```python
from build123d import *

# Parameters (mm, degrees)
SKETCH_2_W               = 22
SKETCH_2_H               = 31.71
EXTRUDE_1_DEPTH          = 22
SKETCH_1_R               = 2.235222544
CUT_EXTRUDE_1_DEPTH      = 38.979461569
CUT_EXTRUDE_2_DEPTH      = 46.024794997
CUT_EXTRUDE_2_DEPTH_BACK = 46.024794997
SKETCH_3_R               = 2.55


with BuildPart() as part:
    # Эскиз2 → Бобышка-Вытянуть1 (new body)
    with BuildSketch(Plane.XY):
        with BuildLine():
            Line((-4.114082915, 26.355832174), (3.885917085, 26.355832174))
            ThreePointArc((3.885917085, 26.355832174), (10.956984897, 23.426899986), (13.885917085, 16.355832174))
            Line((13.885917085, 16.355832174), (13.885917085, -17.554167826))
            ThreePointArc((13.885917085, -17.554167826), (10.956984897, -24.625235638), (3.885917085, -27.554167826))
            Line((3.885917085, -27.554167826), (-4.114082915, -27.554167826))
            ThreePointArc((-4.114082915, -27.554167826), (-11.185150727, -24.625235638), (-14.114082915, -17.554167826))
            Line((-14.114082915, -17.554167826), (-14.114082915, 16.355832174))
            ThreePointArc((-14.114082915, 16.355832174), (-11.185150727, 23.426899986), (-4.114082915, 26.355832174))
        make_face()
        with Locations((-0.114082915, -0.599167826)):
            Rectangle(SKETCH_2_W, SKETCH_2_H, mode=Mode.SUBTRACT)
    extrude(amount=EXTRUDE_1_DEPTH)

    # Эскиз1 → Вырез-Вытянуть1 (cut, through all)
    with BuildSketch(Plane.XY):
        with Locations((-0.114082915, 19.805832174)):
            Circle(SKETCH_1_R)
        with Locations((-0.114082915, -21.004167826)):
            Circle(SKETCH_1_R)
    extrude(amount=CUT_EXTRUDE_1_DEPTH, mode=Mode.SUBTRACT)

    # Эскиз3 → Вырез-Вытянуть2 (cut, two sides: drawn at the far end of the back side and taken through both)
    with BuildSketch(Plane(origin=(13.885917085, 0, 0), x_dir=(0, 0, -1), z_dir=(1, 0, 0)).offset(-CUT_EXTRUDE_2_DEPTH_BACK)):
        with Locations(Location((-11, 2.255832174, 0), (0, 0, 270))):
            Circle(SKETCH_3_R)
    extrude(amount=CUT_EXTRUDE_2_DEPTH + CUT_EXTRUDE_2_DEPTH_BACK, mode=Mode.SUBTRACT)


solid = part.part
```
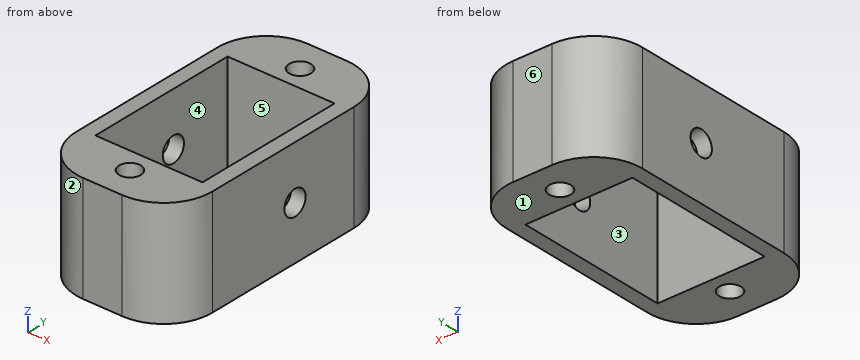
Geometry: final body of the model. Coordinates: model frame, mm. Face numbers are marked on the shaded views. A direction names the side the tool comes from. Round coordinates to 2 decimals unless told otherwise and drop trailing zeros. Loops run counter-clockwise (first coordinate to the right, second up) from the corner with the lowest first, then second, coordinate; pieces in that order, holes last. Notation, with made-up numbers: (42, 39.5) -> (86, 39.5) arc R3 ccw to (86, 43.5) -> close; hole circle Ø3 at (-12, 3.5). An arc over 180 degrees is marked (long way). Use one line per item in the form item = value. Start each with the question number.
1) Access query for the marked faces 5 and 6. Directions: +Z, -Z, +X, -X, +Y, -Y. A direction counts if a zero-diameter tool reaches every point of the face in a straight line with its end or side. Return the directions, or none.
2) Section A-A on y = -2. Output: boundary loops of the cut face in (x, z), then the cut area to 3 significant figures.
3) Section C-C on z = 11. Output: boundary loops of the cut face in (x, y), then the cut area to 3 significant figures.
4) Section D-D on x = -5.5. Output: boundary loops of the cut face in (y, z).
5) First-contact query: P1, Ø1.5, axis at y = -21, z = 3, coming from the -X side. Flat tip, straight axial feed; report the tip coordinate or a pass-through.
6) Draft query along Y for the marked faces 1, 2, 3 and 4. Return one class per face: released by +Y, released by -Y, zero draft, split by the parting line, or undercut.
7) Line query: L1, parallel to X at y = 7, z = 10; L2, parallel to Y at x = -0.5, z = 20.25; L3, parallel to Y at x = 3.5, z = 15. Output: solid intervals per line, ascending.
8) Section B-B on x = -1.5. Output: boundary loops of the cut face in (y, z).
Response:
q1.face_5 = +Z, -Z
q1.face_6 = +Z, -Z, +X, -X, +Y
q2.outline = (-14.11, 0) -> (-11.11, 0) -> (-11.11, 22) -> (-14.11, 22) -> close; (10.89, 0) -> (13.89, 0) -> (13.89, 22) -> (10.89, 22) -> close
q2.area = 132 mm^2
q3.outline = (-14.11, -17.55) arc R10 ccw to (-4.11, -27.55) -> (3.89, -27.55) arc R10 ccw to (13.89, -17.55) -> (13.89, -0.29) -> (10.89, -0.29) -> (10.89, -16.45) -> (-11.11, -16.45) -> (-11.11, -0.29) -> (-14.11, -0.29) -> close; (-14.11, 4.81) -> (-11.11, 4.81) -> (-11.11, 15.26) -> (10.89, 15.26) -> (10.89, 4.81) -> (13.89, 4.81) -> (13.89, 16.36) arc R10 ccw to (3.89, 26.36) -> (-4.11, 26.36) arc R10 ccw to (-14.11, 16.36) -> close; hole circle Ø4.47 at (-0.11, -21); hole circle Ø4.47 at (-0.11, 19.81)
q3.area = 664 mm^2
q4.outline = (-27.46, 0) -> (-16.45, 0) -> (-16.45, 22) -> (-27.46, 22) -> close; (15.26, 0) -> (26.26, 0) -> (26.26, 22) -> (15.26, 22) -> close
q5.P1 = -13.74
q6.face_1 = zero draft
q6.face_2 = released by -Y
q6.face_3 = undercut
q6.face_4 = undercut
q7.L1 = -14.11 to -11.11, 10.89 to 13.89
q7.L2 = -27.55 to -23.21, -18.8 to -16.45, 15.26 to 17.6, 22.01 to 26.36
q7.L3 = -27.55 to -16.45, 15.26 to 26.36
q8.outline = (-27.55, 0) -> (-22.76, 0) -> (-22.76, 22) -> (-27.55, 22) -> close; (-19.25, 0) -> (-16.45, 0) -> (-16.45, 22) -> (-19.25, 22) -> close; (15.26, 0) -> (18.05, 0) -> (18.05, 22) -> (15.26, 22) -> close; (21.56, 0) -> (26.36, 0) -> (26.36, 22) -> (21.56, 22) -> close
